```python
from build123d import *

# Parameters (mm, degrees)
BOSS_EXTRUDE1_DEPTH = 14
SKETCH3_R           = 11.3
SKETCH3_R_2         = 3.6
SKETCH3_R_3         = 3.65
SKETCH3_R_4         = 7.25
CUT_EXTRUDE1_DEPTH  = 14


with BuildPart() as part:
    # Sketch2 → Boss-Extrude1 (new body)
    with BuildSketch(Plane.XY):
        Polygon((-56.968136793, -20), (-56.968136793, 20), (6.031863207, 20), (6.031863207, 40), (58.031863207, 40), (58.031863207, 20), (308.031863207, 20), (308.031863207, 40), (360.031863207, 40), (360.031863207, 20), (423.031863207, 20), (423.031863207, -20), (360.031863207, -20), (360.031863207, -40), (308.031863207, -40), (308.031863207, -20), (58.031863207, -20), (58.031863207, -40), (6.031863207, -40), (6.031863207, -20), align=None)
    extrude(amount=BOSS_EXTRUDE1_DEPTH)

    # Sketch3 → Cut-Extrude1 (cut)
    with BuildSketch(Plane.XY.offset(14)):
        with Locations((-20.968136793, 0)):
            Circle(SKETCH3_R)
        with Locations((-46.968136793, 12.35)):
            Circle(SKETCH3_R_2)
        with Locations((0.031863207, 12.35)):
            Circle(SKETCH3_R_2)
        with Locations(Location((0.031863207, -12.35, 0), (0, 0, 180))):
            Circle(SKETCH3_R_2)
        with Locations(Location((-46.968136793, -12.35, 0), (0, 0, 180))):
            Circle(SKETCH3_R_2)
        with Locations((31.531863207, 25)):
            Circle(SKETCH3_R_3)
        with Locations(Location((31.531863207, -25, 0), (0, 0, 180))):
            Circle(SKETCH3_R_3)
        with Locations((83.031863207, 0)):
            Circle(SKETCH3_R_4)
        with Locations((123.031863207, 0)):
            Circle(SKETCH3_R_4)
        with Locations(Location((283.031863207, 0, 0), (0, 0, 180))):
            Circle(SKETCH3_R_4)
        with Locations(Location((243.031863207, 0, 0), (0, 0, 180))):
            Circle(SKETCH3_R_4)
        with Locations((334.531863207, -25)):
            Circle(SKETCH3_R_3)
        with Locations(Location((334.531863207, 25, 0), (0, 0, 180))):
            Circle(SKETCH3_R_3)
        with Locations((366.031863207, -12.35)):
            Circle(SKETCH3_R_2)
        with Locations(Location((366.031863207, 12.35, 0), (0, 0, 180))):
            Circle(SKETCH3_R_2)
        with Locations(Location((387.031863207, 0, 0), (0, 0, 180))):
            Circle(SKETCH3_R)
        with Locations((413.031863207, -12.35)):
            Circle(SKETCH3_R_2)
        with Locations(Location((413.031863207, 12.35, 0), (0, 0, 180))):
            Circle(SKETCH3_R_2)
    extrude(amount=-CUT_EXTRUDE1_DEPTH, mode=Mode.SUBTRACT)


solid = part.part
```
CAD build for the part. Positions are in the model's coordinates, mm. A direction names the side the tool comes from. Coordinates: 2 decimals unless noted, no trailing zeros. Order: outer loops, then holes, each group sorted by start corner. A loop starts at its lowest first (then second) coordinate and runs counter-clockwise, first axis right, second up.
(1) Saw through at D-D, the plane x = 137. Write the cut outline in (y, z), and give its area (3 significant figures).
Solution:
outline: (-20, 0) - (20, 0) - (20, 14) - (-20, 14) - close
area: 560 mm2
(2) Mould opens along X. For faces 1 (the face through (6.032, -30, 7)), 2 (the face through (308.032, 30, 7)), 3 (the face through (186, 1, 14)) say: released by +X, released by -X, zero draft, split by the parting line, or undercut.
Solution:
face 1: released by -X
face 2: undercut
face 3: zero draft
(3) Pin check, flat tips, straight feed: pin 1 Ø6 at (x, y) = (413.03, -12.35) entering from -Z; pin 2 Ø4 at (y, z) = (26, 4) entering from +X; pin 3 Ø4 at (y, z) = (25, 10) entering from -X. Stop position of each tip, or through.
Solution:
pin 1: passes through
pin 2: stops at x = 360.03
pin 3: stops at x = 6.03
(4) Drill centre lines: L1, parallel to X at y = -13, z = 10; L2, parallel to X at y = 22, z = 4.5; L3, parallel to Y at x = -28, z = 11. Where is each one in solid material? Low to high.
Solution:
L1: x = -56.97 to -50.51, -43.43 to -3.51, 3.57 to 362.49, 369.57 to 409.49, 416.57 to 423.03
L2: x = 6.03 to 29.45, 33.61 to 58.03, 308.03 to 332.45, 336.61 to 360.03
L3: y = -20 to -8.85, 8.85 to 20
(5) Which spindle directions (+Z, -Z, +X, -X, +Y, -Y) get a long thin tool onto all of the face, cutting with end or side? Do faces 4 (the face through (-25, -20, 7)), 5 (the face through (181, 20, 7)), 6 (the face through (392, -20, 7)), 7 (the face through (58.032, -30, 7)). Say none if no direction does.
Solution:
face 4: +Z, -Z, -X, -Y
face 5: +Z, -Z, +Y
face 6: +Z, -Z, +X, -Y
face 7: +Z, -Z, -Y
(6) Saw through at B-B, the plane y = 0. Write the cut outline in (x, z), and give its area (3 significant figures).
Solution:
outline: (-56.97, 0) - (-32.27, 0) - (-32.27, 14) - (-56.97, 14) - close; (-9.67, 0) - (75.78, 0) - (75.78, 14) - (-9.67, 14) - close; (90.28, 0) - (115.78, 0) - (115.78, 14) - (90.28, 14) - close; (130.28, 0) - (235.78, 0) - (235.78, 14) - (130.28, 14) - close; (250.28, 0) - (275.78, 0) - (275.78, 14) - (250.28, 14) - close; (290.28, 0) - (375.73, 0) - (375.73, 14) - (290.28, 14) - close; (398.33, 0) - (423.03, 0) - (423.03, 14) - (398.33, 14) - close
area: 5,280 mm2
(7) Saw through at A-A, the plane y = -34.5. Write the cut outline in (x, z).
Solution:
outline: (6.03, 0) - (58.03, 0) - (58.03, 14) - (6.03, 14) - close; (308.03, 0) - (360.03, 0) - (360.03, 14) - (308.03, 14) - close
(8) Saw through at C-C, the plane z = 5.25. Count the separate pieces of the cut face and the enclosed holes in it, and give its area (3 significant figures).
Solution:
separate pieces: 1
enclosed holes: 18
area: 21,400 mm2
